The model under review builds one solid part; all positions refer to its coordinate system, in mm. Give positions to 0.01 mm unless a question says otherwise; leave off trailing zeros. Write each loop counter-clockwise with the first axis right and the second up, starting at its lowest first coordinate (ties: lowest second). Pieces come first, ordered by that corner, then holes. Notation, with made-up numbers: (46.25, 69.5) - (101.25, 69.5) arc R15 cw to (101.25, 98.5) - close; hole circle Ø9 at (-27, 58). An arc over 180 degrees is marked (long way). Write item = value, one per line.
```python
from build123d import *

# Parameters (mm, degrees)
SKETCH2_R               = 10
BOSS_EXTRUDE1_DEPTH     = 2.5
CUT_EXTRUDE1_DEPTH      = 1
CUT_EXTRUDE1_DEPTH_BACK = 6
BOSS_EXTRUDE2_REACH     = 32
SKETCH4_R               = 2.5


with BuildPart() as part:
    # Sketch2 → Boss-Extrude1 (new body, symmetric)
    with BuildSketch(Plane(origin=(0, 0, 0), x_dir=(0, 0, -1), z_dir=(1, 0, 0))):
        Circle(SKETCH2_R)
    extrude(amount=BOSS_EXTRUDE1_DEPTH, both=True)

    # Sketch3 → Cut-Extrude1 (cut, two sides)
    with BuildSketch(Plane(origin=(2.5, 0, 0), x_dir=(0, 0, -1), z_dir=(1, 0, 0))) as cut_extrude1_sk:
        with BuildLine():
            Line((0, 5), (0, 10))
            ThreePointArc((0, 10), (-10, 0), (0, -10))
            Line((0, -10), (0, -5))
            ThreePointArc((0, -5), (5, 0), (0, 5))
        make_face()
    extrude(amount=CUT_EXTRUDE1_DEPTH, mode=Mode.SUBTRACT)
    extrude(cut_extrude1_sk.sketch, amount=-CUT_EXTRUDE1_DEPTH_BACK, mode=Mode.SUBTRACT)

    # Sketch4 → Boss-Extrude2 (add, up to next)
    with BuildSketch(Plane(origin=(0, 0, -30), x_dir=(-1, 0, 0), z_dir=(0, 0, -1)), mode=Mode.PRIVATE) as boss_extrude2_sk1:
        Circle(SKETCH4_R)
    boss_extrude2_tool1 = extrude(boss_extrude2_sk1.sketch, amount=-BOSS_EXTRUDE2_REACH, mode=Mode.PRIVATE) - part.part
    add(boss_extrude2_tool1.solids().sort_by_distance((0, 0, -30))[0])


solid = part.part
```
1. Take a section at A-A on x = 0. Give the boundary of the cut face in (y, z), and give its area (3 significant figures).
Findings below:
outline = (-10, 0) arc R10 ccw to (-2.5, -9.68) - (-2.5, -30) - (2.5, -30) - (2.5, -9.68) arc R10 ccw to (10, 0) - (5, 0) arc R5 cw to (-5, 0) - close
area = 218 mm²
2. For line 1 (Y direction, x = -0.05, z = -25.5); line 2 (Z direction, x = 2.1, y = -3); line 3 (Y direction, x = -0.65, z = -16.5), list the stretches that pass through material, from the lowest coordinate up. Write a range as from..to.
Findings below:
line_1 = -2.5..2.5
line_2 = -9.54..-4
line_3 = -2.41..2.41
3. Insertion check: P1, Ø3, axis at x = 0, z = -27, coming from the +Y side; P2, Ø1, axis at y = -1, z = -13.5, coming from the -X side; P3, Ø1, axis at x = 2, z = -10.5, coming from the -Y side. Each pin has a flat end and moves straight along its axis. Give the tip position at first contact, or say it passes through.
Findings below:
P1 = 2.5
P2 = -2.45
P3 = -2
4. Take a section at B-B on z = -4.5. Give the boundary of the cut face in (x, y).
Findings below:
outline = (-2.5, -8.93) - (2.5, -8.93) - (2.5, -2.18) - (-2.5, -2.18) - close; (-2.5, 2.18) - (2.5, 2.18) - (2.5, 8.93) - (-2.5, 8.93) - close
5. Draft analysis for pull direction Y (two halves, no side actions). For faces 1 (the cylindrical face through (0, 8, -6)), 2 (the cylindrical face through (-2.385, 0.751, -19.983)), 3 (the flat face through (-2.5, 0, -6)), 4 (the cylindrical face through (0, 0, -5)), state which applies: +Y half, -Y half, draft (parallel to the pull), parting line (faces both ways), or undercut.
Findings below:
face_1 = +Y half
face_2 = parting line
face_3 = draft
face_4 = undercut
6. Take a section at D-D on z = -17. Give the boundary of the cut face in (x, y).
Findings below:
outline = circle Ø5 at (0, 0)
7. Take a section at C-C on y = 1.25. Give the boundary of the cut face in (x, z), and give its area (3 significant figures).
Findings below:
outline = (-2.5, -9.92) - (-2.17, -9.92) - (-2.17, -30) - (2.17, -30) - (2.17, -9.92) - (2.5, -9.92) - (2.5, -4.84) - (-2.5, -4.84) - close
area = 112 mm²
